Build history of the part. All positions in model axes, mm. A direction names the side the tool comes from. Round coordinates to 2 decimals unless told otherwise and drop trailing zeros. Write each loop counter-clockwise with the first axis right and the second up, starting at its lowest first coordinate (ties: lowest second). Pieces come first, ordered by that corner, then holes. Notation, with made-up numbers: M -19.5,75 L 19.5,75 A34 ccw 19.5,113 Z; hole C 16.25,39.5 d3. An arc over 180 degrees is marked long. Write item = value, one per line. Start each with the question number.
Q1. Tool access for faces 1 (the cylindrical face through (-2.75, -1.34, -12.4)), 2 (the cylindrical face through (-3.27, -0.39, 7.25)), 3 (the cylindrical face through (2.75, 0.96, -12.4)): list every direction of +Z, -Z, +X, -X, +Y, -Y with a clear straight run to the whole face (end or side of a thin tool).
Q2. Drop flat-ended pins along their axis: P1, Ø7.5, axis at x = -8.91, z = 0, coming from the -Y side; P2, Ø1, axis at y = -0.5, z = -5, coming from the +X side; P3, Ø5.5, axis at x = -6.3, z = 6.3, coming from the -Y side; P4, Ø1, axis at x = -7, y = 1, coming from the +Z side. Give the stop position or say it passes through.
Q3. Probe L1, parallel to Z at x = 0, y = 0.4; L2, parallel to Z at x = 0, y = -0.3 (3 decimals); L3, parallel to Z at x = -5.5, y = -0.5. List the from-to ranges inside material, lowest first.
Q4. Band-saw the part on B-B on z = -2.5. State how many separate pieces and enclosed holes the cut face has, plus the area to 3 significant figures.
Q5. Band-saw the part on A-A on x = 0. Write the cut outline in (y, z) (1 decimal).
Q6. Pull direction X, two halves, no side cores. Call faces 4 (the flat face through (-11, -1.588, 7)), 5 (the flat face through (0, 0.317, -3)), 6 (the cylindrical face through (-3.441, -0.004, -15.497)): released by +X, released by -X, zero draft, split by the parting line, or undercut.
```python
from build123d import *

# Parameters (mm, degrees)
F0_R     = 15.875
F1_DEPTH = 1.5875
F2_R     = 12.7
F3_DEPTH = 0.508
F4_R     = 12.7
F5_DEPTH = 1.27
F6_R     = 1.27
F7_DEPTH = 2.668
F8_R     = 3.175
F9_DEPTH = 2.668
F10_R    = 1.27


with BuildPart() as f1:
    # F0 (on Front) → F1 (new body, symmetric)
    with BuildSketch(Plane.XZ):
        Circle(F0_R)
    extrude(amount=F1_DEPTH, both=True)

    # F2 (on face) → F3 (cut)
    with BuildSketch(Plane.XZ.offset(1.5875)):
        Circle(F2_R)
    extrude(amount=-F3_DEPTH, mode=Mode.SUBTRACT)

    # F4 (on face) → F5 (cut)
    with BuildSketch(Plane(origin=(0, 1.5875, 0), x_dir=(-1, 0, 0), z_dir=(0, 1, 0))):
        Circle(F4_R)
    extrude(amount=-F5_DEPTH, mode=Mode.SUBTRACT)

    # F6 (on face) → F7 (cut, through all)
    with BuildSketch(Plane.XZ.offset(1.0795)):
        Circle(F6_R)
    extrude(amount=-F7_DEPTH, mode=Mode.SUBTRACT)

    # F8 (on face) → F9 (cut, through all)
    with BuildSketch(Plane.XZ.offset(1.0795)):
        with Locations((0, 8.9109085647)):
            Circle(F8_R)
        with Locations((-6.3009638726, 6.3009638726)):
            Circle(F8_R)
        with Locations((-8.9109085647, 0)):
            Circle(F8_R)
        with Locations((-6.3009638726, -6.3009638726)):
            Circle(F8_R)
        with Locations((0, -8.9109085647)):
            Circle(F8_R)
        with Locations((6.3009638726, -6.3009638726)):
            Circle(F8_R)
        with Locations((8.9109085647, 0)):
            Circle(F8_R)
        with Locations((6.3009638726, 6.3009638726)):
            Circle(F8_R)
    extrude(amount=-F9_DEPTH, mode=Mode.SUBTRACT)

    # F10
    f10_edges = [f1.edges().sort_by_distance(p)[0] for p in [
        (-15.875, -1.5875, 0),
        (-15.875, 1.5875, 0),
        (15.875, 0, 0),
    ]]
    fillet(f10_edges, radius=F10_R)


solid = f1.part
```
Conclusion:
q1.face_1 = -Y
q1.face_2 = +Y, -Y
q1.face_3 = +Y
q2.P1 = -1.08
q2.P2 = 15.22
q2.P3 = through
q2.P4 = 14.37
q3.L1 = -15.87 to -12.7, 12.7 to 15.87
q3.L2 = -15.875 to -12.086, -5.736 to -1.27, 1.27 to 5.736, 12.086 to 15.875
q3.L3 = -14.88 to -9.37, -3.23 to 3.23, 9.37 to 14.88
q4.separate_pieces = 3
q4.enclosed_holes = 0
q4.area = 42.9 mm^2
q5.outline = M -1.6,-14.6 A1.3 ccw -0.3,-15.9 L 0.3,-15.9 A1.3 ccw 1.6,-14.6 L 1.6,-12.7 L 0.3,-12.7 L 0.3,-12.1 L -1.1,-12.1 L -1.1,-12.7 L -1.6,-12.7 Z; M -1.6,12.7 L -1.1,12.7 L -1.1,12.1 L 0.3,12.1 L 0.3,12.7 L 1.6,12.7 L 1.6,14.6 A1.3 ccw 0.3,15.9 L -0.3,15.9 A1.3 ccw -1.6,14.6 Z; M -1.1,-5.7 L 0.3,-5.7 L 0.3,-1.3 L -1.1,-1.3 Z; M -1.1,1.3 L 0.3,1.3 L 0.3,5.7 L -1.1,5.7 Z
q6.face_4 = zero draft
q6.face_5 = undercut
q6.face_6 = split by the parting line
